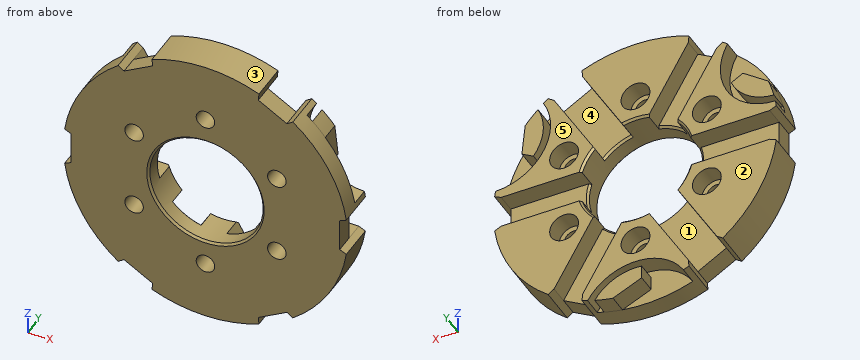
```python
from build123d import *

# Parameters (mm, degrees)
SKETCH1_R                               = 69
BOSS_EXTRUDE1_DEPTH                     = 18
SKETCH2_R                               = 27.5
CUT_EXTRUDE1_DEPTH                      = 100.227012451
CUT_EXTRUDE2_DEPTH                      = 9
CUT_EXTRUDE3_START                      = -9
CUT_EXTRUDE3_DEPTH                      = 9
CIRPATTERN1_COUNT                       = 6
CUT_EXTRUDE4_START                      = -9
SKETCH5_R                               = 27
CUT_EXTRUDE4_DEPTH                      = 9
CIRPATTERN2_COUNT                       = 3
CBORE_FOR_M5_HEX_HEAD_BOLT1_D           = 9
CBORE_FOR_M5_HEX_HEAD_BOLT1_CBORE_D     = 14
CBORE_FOR_M5_HEX_HEAD_BOLT1_CBORE_DEPTH = 9
CIRPATTERN3_COUNT                       = 6
CHAMFER1_SIZE                           = 1


with BuildPart() as part:
    # Sketch1 → Boss-Extrude1 (new body)
    with BuildSketch(Plane(origin=(0, 0, 0), x_dir=(1, 0, 0), z_dir=(0, 1, 0))):
        with Locations(Location((0, 0, 0), (0, 0, 270))):
            Circle(SKETCH1_R)
    extrude(amount=BOSS_EXTRUDE1_DEPTH)

    # Sketch2 → Cut-Extrude1 (cut, through all)
    with BuildSketch(Plane(origin=(0, 18, 0), x_dir=(1, 0, 0), z_dir=(0, 1, 0))):
        with Locations(Location((0, 0, 0), (0, 0, 270))):
            Circle(SKETCH2_R)
    extrude(amount=-CUT_EXTRUDE1_DEPTH, mode=Mode.SUBTRACT)

    # Sketch3 → Cut-Extrude2 (cut)
    with BuildSketch(Plane(origin=(0, 18, 0), x_dir=(1, 0, 0), z_dir=(0, 1, 0))):
        with BuildLine():
            Line((-39.506230912, 52.426799156), (-20.083525347, 18.785686296))
            ThreePointArc((-20.083525347, 18.785686296), (-13.75, 23.815698604), (-6.227118887, 26.785686296))
            Line((-6.227118887, 26.785686296), (-25.649824452, 60.426799156))
            Line((-25.649824452, 60.426799156), (-25.956463368, 63.931698002))
            ThreePointArc((-25.956463368, 63.931698002), (-34.5, 59.755752861), (-42.388242893, 54.44480567))
            Line((-42.388242893, 54.44480567), (-39.506230912, 52.426799156))
        make_face()
    cut_extrude2 = extrude(amount=-CUT_EXTRUDE2_DEPTH, mode=Mode.SUBTRACT)

    # Sketch4 → Cut-Extrude3 (cut)
    with BuildSketch(Plane(origin=(0, 9, 0), x_dir=(1, 0, 0), z_dir=(0, 1, 0)).offset(CUT_EXTRUDE3_START)):
        with BuildLine():
            Line((-39.506230912, 52.426799156), (-25.649824452, 60.426799156))
            Line((-25.649824452, 60.426799156), (-25.956463368, 63.931698002))
            ThreePointArc((-25.956463368, 63.931698002), (-34.5, 59.755752861), (-42.388242893, 54.44480567))
            Line((-42.388242893, 54.44480567), (-39.506230912, 52.426799156))
        make_face()
    cut_extrude3 = extrude(amount=CUT_EXTRUDE3_DEPTH, mode=Mode.SUBTRACT)

    # CirPattern1: Cut-Extrude2, Cut-Extrude3 ×6 about axis
    cirpattern1_axis = Axis((0, 0, 0), (0, 1, 0))
    add([cut_extrude2.rotate(cirpattern1_axis, i * 360 / CIRPATTERN1_COUNT) for i in range(1, CIRPATTERN1_COUNT)], mode=Mode.SUBTRACT)
    add([cut_extrude3.rotate(cirpattern1_axis, i * 360 / CIRPATTERN1_COUNT) for i in range(1, CIRPATTERN1_COUNT)], mode=Mode.SUBTRACT)

    # Sketch5 → Cut-Extrude4 (cut)
    with BuildSketch(Plane(origin=(0, 18, 0), x_dir=(1, 0, 0), z_dir=(0, 1, 0)).offset(CUT_EXTRUDE4_START)):
        with Locations((-68.199500548, -39.375)):
            Circle(SKETCH5_R)
        with BuildLine():
            Line((-52.130681517, -33.561764622), (-46.514419424, -30.319214191))
            ThreePointArc((-46.514419424, -30.319214191), (-54.735535714, -20.114375634), (-67.143353435, -15.898744905))
            ThreePointArc((-67.143353435, -15.898744905), (-65.948291272, -20.29341958), (-64.465924789, -24.599685792))
            Line((-64.465924789, -24.599685792), (-52.130681517, -33.561764622))
        make_face(mode=Mode.SUBTRACT)
    cut_extrude4 = extrude(amount=CUT_EXTRUDE4_DEPTH, mode=Mode.SUBTRACT)

    # CirPattern2: Cut-Extrude4 ×3 about axis
    cirpattern2_axis = Axis((0, 0, 0), (0, 1, 0))
    for i in range(1, CIRPATTERN2_COUNT):
        add(cut_extrude4.rotate(cirpattern2_axis, i * 360 / CIRPATTERN2_COUNT), mode=Mode.SUBTRACT)

    # CBORE for M5 Hex Head Bolt1 (through all)
    with Locations(Plane(origin=(0, 18, -40), x_dir=(0, 0, 1), z_dir=(0, 1, 0))):
        with Locations((0, 0)):
            cbore_for_m5_hex_head_bolt1 = CounterBoreHole(CBORE_FOR_M5_HEX_HEAD_BOLT1_D / 2, CBORE_FOR_M5_HEX_HEAD_BOLT1_CBORE_D / 2, CBORE_FOR_M5_HEX_HEAD_BOLT1_CBORE_DEPTH)

    # CirPattern3: CBORE for M5 Hex Head Bolt1 ×6 about axis
    cirpattern3_axis = Axis((0, 0, 0), (0, 1, 0))
    for i in range(1, CIRPATTERN3_COUNT):
        add(cbore_for_m5_hex_head_bolt1.rotate(cirpattern3_axis, i * 360 / CIRPATTERN3_COUNT), mode=Mode.SUBTRACT)

    # Chamfer1
    chamfer1_edges = [part.edges().sort_by_distance(p)[0] for p in [
        (-23.815698604, 18, -13.75),
        (-27.5, 9, 0),
        (-13.75, 9, -23.815698604),
        (-23.815698604, 18, 13.75),
        (3.133977253, 18, 27.320837955),
        (23.815698604, 18, 13.75),
        (23.815698604, 18, -13.75),
        (0, 18, -27.5),
        (0, 0, -27.5),
        (13.75, 9, -23.815698604),
        (27.5, 9, 0),
        (13.75, 9, 23.815698604),
        (-13.75, 9, 23.815698604),
    ]]
    chamfer(chamfer1_edges, length=CHAMFER1_SIZE)


solid = part.part
```
Can you work these out from the model? Positions are in its coordinate system, mm. Face numbers are marked on the shaded views. A direction names the side the tool comes from. Round coordinates to 2 decimals unless told otherwise and drop trailing zeros. Order: outer loops, then holes, each group sorted by start corner. A loop starts at its lowest first (then second) coordinate and runs counter-clockwise, first axis right, second up.
(1) If I drill on L1, parallel to X at y = 14.5, z = -59; L2, parallel to X at y = 11.5, z = -20; L3, parallel to X at y = 3.5, z = -20, over which ranges is the centre line in solid material (lowest first)?
Results are:
L1: x = -24.83 to -18.41, -3 to 12.74, 18.41 to 24.83
L2: x = -66.04 to -41.64, -27.64 to -20.78, 20.78 to 27.64, 41.64 to 66.04
L3: x = -66.04 to -39.14, -30.14 to -18.87, 18.87 to 30.14, 39.14 to 66.04
(2) If we section it at B-B (y = 3.5): Count the separate pieces of the cut face and the enclosed holes in it, plus the area to 3 significant figures.
Results are:
separate pieces: 1
enclosed holes: 7
area: 11,800 mm2
(3) I'm going to push flat-ended pins straight in: pin 1 (3 mm diameter, centred on x = 29, y = 2, fed in from -Z); pin 2 (5 mm diameter, centred on x = -37.5, z = 2, fed in from +Y); pin 3 (5 mm diameter, centred on x = -38, y = 13, fed in from -Z). Where does each tip first touch, or does it pass through?
Results are:
pin 1: stops at z = -59.36
pin 2: stops at y = 9
pin 3: stops at z = -53.12
(4) On a 3-axis mill with a long thin cutter (end or side, diameter ignored), from which of +Z, -Z, +X, -X, +Y, -Y can I reach the whole of each face in a straight line? I mean the marked faces 1 and 2. Say none if no direction works.
Results are:
face 1: +Y
face 2: +Z, -Z, +X, -X, +Y
(5) If we section it at A-A (z = 0): Please give me the cut outline in (x, y), plus the area to 3 significant figures.
Results are:
outline: (-65.16, 0) - (-28.5, 0) - (-27.5, 1) - (-27.5, 8) - (-28.5, 9) - (-65.16, 9) - close; (27.5, 1) - (28.5, 0) - (65.16, 0) - (65.16, 9) - (28.5, 9) - (27.5, 8) - close
area: 676 mm2
(6) If we section it at C-C (x = -54.5): Please give me the cut outline in (y, z), plus the area to 3 significant figures.
Results are:
outline: (0, -42.32) - (18, -42.32) - (18, -8) - (9, -8) - (9, 8) - (18, 8) - (18, 16.11) - (9, 16.11) - (9, 20.28) - (18, 20.28) - (18, 31.84) - (9, 31.84) - (9, 42.32) - (0, 42.32) - close
area: 1,250 mm2
(7) We'd pull the mould along Z, two halves only. Please class the marked faces 3, 4 and 5: +Z half, -Z half, draft (parallel to the pull), parting line (faces both ways), or undercut.
Results are:
face 3: +Z half
face 4: undercut
face 5: draft
